Autodesk Inventor part; units mm, degrees
ref_plane "YZ Plane" through (0, 0, 0) normal (1, 0, 0) x (0, 1, 0)
ref_plane "XZ Plane" through (0, 0, 0) normal (0, 1, 0) x (-1, 0, 0)
ref_plane "XY Plane" through (0, 0, 0) normal (0, 0, 1) x (1, 0, 0)
sketch "Sketch1" plane through (0, 0, 0) normal (0, 0, 1) x (1, 0, 0)
  line L0 (0, 0) -> (88.9, 0)
  line L1 (88.9, 0) -> (88.9, 63.5)
  line L2 (88.9, 63.5) -> (0, 63.5)
  line L3 (0, 63.5) -> (0, 0)
  dimension "d0" = 88.9
  dimension "d1" = 63.5
extrude "Extrusion1" add sketch "Sketch1" along normal blind 3.175
sketch "Sketch2" plane through (0, 0, 3.175) normal (0, 0, 1) x (1, 0, 0)
  line L0 (16.891, 13.97) -> (72.009, 13.97)
  line L1 (72.009, 13.97) -> (72.009, 49.53)
  line L2 (72.009, 49.53) -> (16.891, 49.53)
  line L3 (16.891, 49.53) -> (16.891, 13.97)
  circle A0 centre (21.971, 43.688) radius 2.0828
  circle A1 centre (66.929, 43.688) radius 2.0828
  circle A2 centre (66.929, 19.812) radius 2.0828
  circle A3 centre (21.971, 19.812) radius 2.0828
  line L4 (29.8704, 19.9898) -> (59.0042, 19.9898)
  line L5 (65.3542, 26.3398) -> (65.3542, 37.5158)
  line L6 (59.0042, 43.8658) -> (29.8704, 43.8658)
  line L7 (23.5204, 37.5158) -> (23.5204, 26.3398)
  arc A4 (29.8704, 43.8658) -> (23.5204, 37.5158) centre (29.8704, 37.5158) ccw
  arc A5 (23.5204, 26.3398) -> (29.8704, 19.9898) centre (29.8704, 26.3398) ccw
  arc A6 (59.0042, 19.9898) -> (65.3542, 26.3398) centre (59.0042, 26.3398) ccw
  arc A7 (65.3542, 37.5158) -> (59.0042, 43.8658) centre (59.0042, 37.5158) ccw
  line L8 (0, 63.5) -> (0, 0)
  line L9 (88.9, 0) -> (88.9, 63.5)
  line L10 (0, 0) -> (88.9, 0)
  line L11 (88.9, 63.5) -> (0, 63.5)
  point P0 (23.5204, 19.9898)
  point P1 (65.3542, 43.8658)
  point P2 (65.3542, 19.9898)
  dimension "d4" = 55.118
  dimension "d5" = 35.56
  dimension "d6" = 4.1656
  dimension "d7" = 5.08
  dimension "d8" = 5.842
  dimension "d9" = 5.842
  dimension "d10" = 5.842
  dimension "d11" = 5.842
  dimension "d12" = 5.08
  dimension "d13" = 5.08
  dimension "d14" = 5.08
  dimension "d15" = 23.876
  dimension "d16" = 41.8338
  dimension "d17" = 1.5748
  dimension "d18" = 0.1778
  dimension "d19" = 6.35
  dimension "d20" = 88.9
  dimension "d21" = 63.5
  dimension "d22" = 13.97
  dimension "d23" = 16.891
extrude "Extrusion2" cut sketch "Sketch2" against normal through all contours A0 | A1 | A2 | A3 | A5 L7 A4 L6 A7 L5 A6 L4
sketch "Sketch4" plane through (0, 0, 3.175) normal (0, 0, 1) x (1, 0, 0)
  line L0 (38.1, 57.15) -> (51.2683, 57.15) construction
  line L1 (51.2683, 57.15) -> (51.2683, 45.6081) construction
  line L2 (51.2683, 45.6081) -> (38.1, 45.6081) construction
  line L3 (38.1, 45.6081) -> (38.1, 57.15) construction
  line L4 (0, 63.5) -> (0, 0)
  line L5 (88.9, 63.5) -> (0, 63.5)
sketch "Sketch5" plane through (0, 0, 0) normal (0, 0, -1) x (-1, 0, 0)
  line L0 (-61.8811, 60.2648) -> (-25.8263, 60.2648) construction
  line L1 (-25.8263, 60.2648) -> (-25.8263, 56.54) construction
  line L2 (-25.8263, 56.54) -> (-61.8811, 56.54) construction
  line L3 (-61.8811, 56.54) -> (-61.8811, 60.2648) construction
  point P0 (0, 0)
sketch "Sketch6" plane through (0, 0, 3.175) normal (0, 0, 1) x (1, 0, 0)
  line L0 (0, 63.5) -> (0, 0)
  circle A0 centre (66.929, 43.688) radius 2.0828
  circle A1 centre (21.971, 19.812) radius 2.0828
  circle A2 centre (21.971, 43.688) radius 2.0828
  circle A3 centre (66.929, 19.812) radius 2.0828
  arc A4 (59.0042, 19.9898) -> (65.3542, 26.3398) centre (59.0042, 26.3398) ccw
  line L1 (59.0042, 19.9898) -> (29.8704, 19.9898)
  arc A5 (23.5204, 26.3398) -> (29.8704, 19.9898) centre (29.8704, 26.3398) ccw
  line L2 (23.5204, 26.3398) -> (23.5204, 37.5158)
  arc A6 (29.8704, 43.8658) -> (23.5204, 37.5158) centre (29.8704, 37.5158) ccw
  line L3 (29.8704, 43.8658) -> (59.0042, 43.8658)
  arc A7 (65.3542, 37.5158) -> (59.0042, 43.8658) centre (59.0042, 37.5158) ccw
  line L4 (65.3542, 37.5158) -> (65.3542, 26.3398)
  line L5 (0, 0) -> (88.9, 0)
  line L6 (88.9, 0) -> (88.9, 63.5)
  line L7 (88.9, 63.5) -> (0, 63.5)
  line L8 (0, 63.5) -> (0, 0)
  point P0 (6.35, 57.15)
  point P1 (82.55, 57.15)
  point P2 (82.55, 6.35)
  point P3 (6.35, 6.35)
  dimension "d57" = 6.35
  dimension "d58" = 6.35
  dimension "d59" = 6.35
  dimension "d60" = 6.35
  dimension "d61" = 6.35
  dimension "d62" = 6.35
  dimension "d63" = 6.35
  dimension "d64" = 6.35
hole "Hole1" at (6.35, 57.15, 3.175) at (6.35, 6.35, 3.175) at (82.55, 6.35, 3.175) at (82.55, 57.15, 3.175) direction (0, 0, -1) diameter 3.302 end through all
thread "Thread9"
thread "Thread10"
thread "Thread11"
thread "Thread12"
equation "\"d9\" = d8"
equation "\"d10\" = d9"
equation "\"d11\" = d8"
equation "\"d12\" = d7"
equation "\"d13\" = d7"
equation "\"d14\" = d7"
equation "\"d22\" = -0.5 * d5 + 0.5 * d21"
equation "\"d23\" = -0.5 * d4 + 0.5 * d20"
properties part number "LFEV2017_TSI_007"
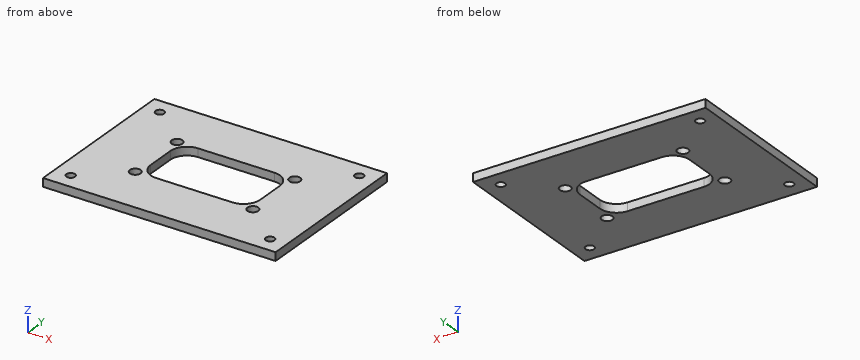
Source: CAD feature listing. Evaluate the final solid. Frame: model axes, mm. Round coordinates to 2 decimals unless told otherwise and drop trailing zeros. Loops run counter-clockwise (first coordinate to the right, second up) from the corner with the lowest first, then second, coordinate; pieces in that order, holes last. Notation, with made-up numbers: M 0,26 L 23,26 A19 ccw 23,43 Z; hole C 8.5,-19 d2. An arc over 180 degrees is marked long. Put each result on its own line as item: value.
(1) Section A-A, the plane x = 6.35. Return loops of the section in (y, z) (3 decimals).
Solutions:
outline: M 0,0 L 4.699,0 L 4.699,3.175 L 0,3.175 Z; M 8.001,0 L 55.499,0 L 55.499,3.175 L 8.001,3.175 Z; M 58.801,0 L 63.5,0 L 63.5,3.175 L 58.801,3.175 Z
(2) Section C-C, the plane x = 41. Return loops of the section in (y, z) (3 decimals).
Solutions:
outline: M 0,0 L 19.99,0 L 19.99,3.175 L 0,3.175 Z; M 43.866,0 L 63.5,0 L 63.5,3.175 L 43.866,3.175 Z
(3) Ray query, line 1 (Y direction, x = 6.35, z = 2.1); line 2 (X direction, y = 6.35, z = 1.7); line 3 (Y direction, x = 35.5, z = 1.8). Return the intervals inside material, ascending. Write a range as [from, to].
Solutions:
line 1: [0, 4.7], [8, 55.5], [58.8, 63.5]
line 2: [0, 4.7], [8, 80.9], [84.2, 88.9]
line 3: [0, 19.99], [43.87, 63.5]
(4) Section D-D, the plane y = 6.35. Return loops of the section in (x, z) (3 decimals).
Solutions:
outline: M 0,0 L 4.699,0 L 4.699,3.175 L 0,3.175 Z; M 8.001,0 L 80.899,0 L 80.899,3.175 L 8.001,3.175 Z; M 84.201,0 L 88.9,0 L 88.9,3.175 L 84.201,3.175 Z
(5) Section B-B, the plane y = 34.5. Return loops of the section in (x, z) (3 decimals).
Solutions:
outline: M 0,0 L 23.52,0 L 23.52,3.175 L 0,3.175 Z; M 65.354,0 L 88.9,0 L 88.9,3.175 L 65.354,3.175 Z
